Here's how the part is built. I have some questions about the finished solid (model axes, mm). Face numbers are marked on the shaded views. A direction names the side the tool comes from. Round coordinates to 2 decimals unless told otherwise and drop trailing zeros. Order: outer loops, then holes, each group sorted by start corner. A loop starts at its lowest first (then second) coordinate and runs counter-clockwise, first axis right, second up. Notation, with made-up numbers: (13, 59.25) - (21, 59.25) arc R26 ccw to (21, 85.25) - close; hole circle Ø2 at (-30.5, 13). An arc over 180 degrees is marked (long way). Answer as a JSON object with one key per item and string values.
```python
from build123d import *

# Parameters (mm, degrees)
BOSS_EXTRUDE1_DEPTH  = 7.5
SKETCH2_R            = 1.6
CUT_EXTRUDE1_DEPTH   = 65.077737633
BOSS_EXTRUDE4_START  = -7.5
BOSS_EXTRUDE4_DEPTH  = 7.5
SKETCH4_R            = 1.6
CUT_EXTRUDE2_DEPTH   = 2.6
SKETCH6_R            = 156.176390482
CUT_EXTRUDE3_DEPTH   = 1
FILLET1_R            = 5
FILLET2_R            = 5
FILLET3_R            = 5
FILLET4_R            = 5
BOSS_EXTRUDE5_DEPTH  = 1.75
MIRROR9_COPY_1_DEPTH = 1.75


with BuildPart() as part:
    # Sketch1 → Boss-Extrude1 (new body)
    with BuildSketch(Plane(origin=(0, 0, 0), x_dir=(1, 0, 0), z_dir=(0, 1, 0))):
        with BuildLine():
            ThreePointArc((-53.020313644, 8), (-50.871094703, 4.253905297), (-50.125, 0))
            ThreePointArc((-50.125, 0), (-49.964111284, 4.012880342), (-49.482477959, 8))
            Line((-49.482477959, 8), (-53.020313644, 8))
        make_face()
        with BuildLine():
            ThreePointArc((-49.482477959, 8), (-49.964111284, 4.012880342), (-50.125, 0))
            Line((-50.125, 0), (-43.319433445, 0))
            ThreePointArc((-43.319433445, 0), (-43.758313694, 4.093048719), (-45.055, 8))
            Line((-45.055, 8), (-49.482477959, 8))
        make_face()
        with BuildLine():
            ThreePointArc((-45.055, 8), (-43.758313694, 4.093048719), (-43.319433445, 0))
            Line((-43.319433445, 0), (-37.555, 0))
            Line((-37.555, 0), (-37.555, 8))
            Line((-37.555, 8), (-45.055, 8))
        make_face()
        with BuildLine():
            ThreePointArc((-48.396817166, 13.048513832), (-49.004703616, 10.538246936), (-49.482477959, 8))
            Line((-49.482477959, 8), (-45.055, 8))
            ThreePointArc((-45.055, 8), (-46.526770878, 10.656074283), (-48.396817166, 13.048513832))
        make_face()
        with BuildLine():
            ThreePointArc((-62.625, 12.5), (-57.321699141, 11.319231423), (-53.020313644, 8))
            Line((-53.020313644, 8), (-49.482477959, 8))
            ThreePointArc((-49.482477959, 8), (-49.004703616, 10.538246936), (-48.396817166, 13.048513832))
            ThreePointArc((-48.396817166, 13.048513832), (-54.853386661, 17.672207732), (-62.625, 19.305566555))
            Line((-62.625, 19.305566555), (-62.625, 12.5))
        make_face()
    boss_extrude1 = extrude(amount=BOSS_EXTRUDE1_DEPTH)

    # Sketch2 → Cut-Extrude1 (cut, through all)
    with BuildSketch(Plane(origin=(0, 0, -8), x_dir=(-1, 0, 0), z_dir=(0, 0, -1))):
        with Locations((41.305, 3.75)):
            Circle(SKETCH2_R)
    cut_extrude1 = extrude(amount=-CUT_EXTRUDE1_DEPTH, mode=Mode.SUBTRACT)

    # Sketch3 → Boss-Extrude4 (add)
    with BuildSketch(Plane(origin=(0, 7.5, 0), x_dir=(1, 0, 0), z_dir=(0, 1, 0)).offset(BOSS_EXTRUDE4_START)):
        with BuildLine():
            ThreePointArc((-62.625, 19.305566555), (-53.806914146, 17.173999589), (-46.936073969, 11.25))
            ThreePointArc((-46.936073969, 11.25), (-25.405775196, 25.617547828), (0, 30.57))
            Line((0, 30.57), (0, 35.57))
            ThreePointArc((0, 35.57), (-32.221430215, 30.937551956), (-62.625, 19.305566555))
        make_face()
    boss_extrude4 = extrude(amount=BOSS_EXTRUDE4_DEPTH)

    # Sketch4 → Cut-Extrude2 (cut)
    with BuildSketch(Plane(origin=(0, 0, -8), x_dir=(-1, 0, 0), z_dir=(0, 0, -1))):
        Polygon((39.735, 1.030680232), (42.875, 1.030680232), (44.445, 3.75), (42.875, 6.469319768), (39.735, 6.469319768), (38.165, 3.75), align=None)
        with Locations((41.305, 3.75)):
            Circle(SKETCH4_R, mode=Mode.SUBTRACT)
    cut_extrude2 = extrude(amount=-CUT_EXTRUDE2_DEPTH, mode=Mode.SUBTRACT)

    # Mirror5: Boss-Extrude4 across plane
    add(boss_extrude4.mirror(Plane(origin=(0, 0, 0), x_dir=(0, 0, 1), z_dir=(1, 0, 0))))

    # Mirror6: Boss-Extrude1 across plane
    add(boss_extrude1.mirror(Plane(origin=(0, 0, 0), x_dir=(0, 0, 1), z_dir=(1, 0, 0))))

    # Mirror7: Cut-Extrude1, Cut-Extrude2 across plane
    add(cut_extrude1.mirror(Plane(origin=(0, 0, 0), x_dir=(0, 0, 1), z_dir=(1, 0, 0))), mode=Mode.SUBTRACT)
    add(cut_extrude2.mirror(Plane(origin=(0, 0, 0), x_dir=(0, 0, 1), z_dir=(1, 0, 0))), mode=Mode.SUBTRACT)

    # Sketch6 → Cut-Extrude3 (cut)
    with BuildSketch(Plane.XY):
        Circle(SKETCH6_R)
    extrude(amount=-CUT_EXTRUDE3_DEPTH, mode=Mode.SUBTRACT)

    # Fillet1
    fillet1_edges = [part.edges().sort_by_distance(p)[0] for p in [
        (-62.625, 3.75, -19.305566555),
    ]]
    fillet(fillet1_edges, radius=FILLET1_R)

    # Fillet2
    fillet2_edges = [part.edges().sort_by_distance(p)[0] for p in [
        (62.625, 3.75, -19.305566555),
    ]]
    fillet(fillet2_edges, radius=FILLET2_R)

    # Fillet3
    fillet3_edges = [part.edges().sort_by_distance(p)[0] for p in [
        (-46.936073969, 3.75, -11.25),
    ]]
    fillet(fillet3_edges, radius=FILLET3_R)

    # Fillet4
    fillet4_edges = [part.edges().sort_by_distance(p)[0] for p in [
        (46.936073969, 3.75, -11.25),
    ]]
    fillet(fillet4_edges, radius=FILLET4_R)

    # Sketch7 → Boss-Extrude5 (add)
    with BuildSketch(Plane(origin=(0, 7.5, 0), x_dir=(1, 0, 0), z_dir=(0, 1, 0))):
        with BuildLine():
            Line((-50.165064206, 1), (-37.555, 1))
            Line((-37.555, 1), (-37.555, 29.44421276))
            ThreePointArc((-37.555, 29.44421276), (-43.910509627, 27.37533218), (-50.165064206, 25.0187846))
            Line((-50.165064206, 25.0187846), (-50.165064206, 1))
        make_face()
    boss_extrude5 = extrude(amount=BOSS_EXTRUDE5_DEPTH)

    # Mirror8: Boss-Extrude5 across plane
    add(boss_extrude5.mirror(Plane.ZX.offset(3.75)))

    # Mirror9: Boss-Extrude5 across plane
    add(boss_extrude5.mirror(Plane(origin=(0, 0, 0), x_dir=(0, 0, 1), z_dir=(1, 0, 0))))

    # Mirror9 copy 1 sketch → Mirror9 copy 1 (add)
    with BuildSketch(Plane(origin=(0, 0, 0), x_dir=(-1, 0, 0), z_dir=(0, -1, 0))):
        with BuildLine():
            Line((-50.165064206, 1), (-37.555, 1))
            Line((-37.555, 1), (-37.555, 29.44421276))
            ThreePointArc((-37.555, 29.44421276), (-43.910509627, 27.37533218), (-50.165064206, 25.0187846))
            Line((-50.165064206, 25.0187846), (-50.165064206, 1))
        make_face()
    extrude(amount=MIRROR9_COPY_1_DEPTH)


solid = part.part
```
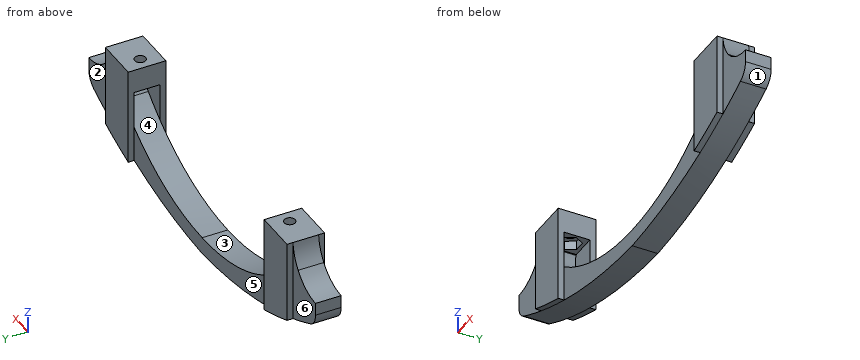
1. Imagine slicing it at C-C (x = -32). List the corners of the cut face in (y, z) for me.
Responses:
{"outline": "(0, -30.99) - (7.5, -30.99) - (7.5, -22.46) - (0, -22.46) - close"}
2. For P1, Ø10, axis at x = -54, z = -13.5, coming from the -Y side; P2, Ø13.5, axis at x = 57.5, z = -10, coming from the +Y side; P3, Ø0.9, axis at y = 8.5, z = -7, coming from the -X side; P4, Ø6, axis at x = 59, z = -11.5, coming from the -Y side, each with a flat end and sliding along its axis, tell me the tip position at first contact or that it passes through.
Responses:
{"P1": "y = -1.75", "P2": "y = 7.5", "P3": "x = -50.17", "P4": "y = 0"}
3. Imagine slicing it at A-A (z = -22). List the corners of the cut face in (x, y) for me (3 decimals), plus the area to 3 significant figures.
Responses:
{"outline": "(-57.129, 0) - (-50.165, 0) - (-50.165, -1.75) - (-37.555, -1.75) - (-37.555, 0) - (-32.832, 0) - (-32.832, 7.5) - (-37.555, 7.5) - (-37.555, 9.25) - (-50.165, 9.25) - (-50.165, 7.5) - (-57.129, 7.5) - close; (32.832, 0) - (37.555, 0) - (37.555, -1.75) - (50.165, -1.75) - (50.165, 0) - (57.129, 0) - (57.129, 7.5) - (50.165, 7.5) - (50.165, 9.25) - (37.555, 9.25) - (37.555, 7.5) - (32.832, 7.5) - close", "area": "453 mm2"}
4. Thinking about a two-plate mould opening in Z: for the marked faces 1, 2 and 3, which applies, pulls with the +Z half, pulls with the -Z half, needs draft (parallel to the pull), parting line crosses it, or undercut?
Responses:
{"face 1": "pulls with the -Z half", "face 2": "needs draft", "face 3": "undercut"}
5. Imagine slicing it at D-D (x = -9.5). List the corners of the cut face in (y, z) for me, plus the area to 3 significant figures.
Responses:
{"outline": "(0, -34.96) - (7.5, -34.96) - (7.5, -29.93) - (0, -29.93) - close", "area": "37.7 mm2"}
6. Imagine slicing it at B-B (x = 41). List the corners of the cut face in (y, z) for me, plus the area to 3 significant figures.
Responses:
{"outline": "(-1.75, -28.36) - (9.25, -28.36) - (9.25, -1) - (5.32, -1) - (5.32, -5.4) - (6.47, -5.4) - (6.47, -8) - (7.5, -8) - (7.5, -16.52) - (0, -16.52) - (0, -8) - (1.03, -8) - (1.03, -5.4) - (2.18, -5.4) - (2.18, -1) - (-1.75, -1) - close", "area": "209 mm2"}
7. For the marked faces 4, 5 and 6, which set-ups out of +Z, -Z, +X, -X, +Y, -Y let a thin tool reach every point of the face, with its end or its side?
Responses:
{"face 4": "none", "face 5": "+Z, -Z, +Y", "face 6": "+Z, -Z, -X, +Y"}
8. If I drill on L1, parallel to X at y = 9, z = -4 (3 decimals); L2, parallel to X at y = 3.5, z = -15 (3 decimals); L3, parallel to Y at x = -27, z = -32, over which ranges is the centre line in solid material (lowest first)? Write a range as [from, to].
Responses:
{"L1": "[-50.165, -37.555], [37.555, 50.165]", "L2": "[-62.625, -42.865], [42.865, 62.625]", "L3": "[0, 7.5]"}
